Could you check a few things on this model? Use its own coordinates, in mm. Coordinates: 2 decimals unless noted, no trailing zeros. Loops run counter-clockwise (first coordinate to the right, second up) from the corner with the lowest first, then second, coordinate; pieces in that order, holes last. Notation, with made-up numbers: (45, -19.75) - (104, -19.75) arc R19 cw to (104, -15.75) - close; hole circle Ø2 at (67.5, -17). An arc over 180 degrees is marked (long way). One line per question, with ' | ' between items. Start each with the question number.
1. I want a section at A-A, the plane y = -55. Write out the boundary of the cut face in (x, z).
2. I want a section at B-B, the plane x = 20.5. Write out the boundary of the cut face in (y, z), then the cut area to 3 significant figures.
3. I want a section at D-D, the plane y = -79.5. Write out the boundary of the cut face in (x, z).
4. Please list where these lines run through material, in increasing order: L1, parallel to Z at x = -4, y = -69.5; L2, parallel to X at y = -117.5, z = -1; L3, parallel to X at y = -47, z = -3.5. Write a range as [from, to].
5. I'm going to push flat-ended pins straight in: P1, Ø12, axis at x = -25.5, y = -16, coming from the +Z side; P2, Ø1.5, axis at y = -92.5, z = -15, coming from the -X side; P3, Ø4.5, axis at y = -27.5, z = -28, coming from the +X side. Where does each tip first touch, or does it pass through?
6. I want a section at C-C, the plane z = -20. Write out the boundary of the cut face in (x, y).
from build123d import *

# Parameters (mm, degrees)
F1_DEPTH = 130
F3_DEPTH = 38


with BuildPart() as f1:
    # F0 (on Front) → F1 (new body)
    with BuildSketch(Plane.XZ):
        with BuildLine():
            ThreePointArc((39.633115, 3.448032), (1.680451, -18.731595), (-40.366885, -31.551968))
            Line((-40.366885, -31.551968), (39.633115, -31.551968))
            Line((39.633115, -31.551968), (39.633115, 3.448032))
        make_face()
    extrude(amount=F1_DEPTH)

    # F2 (on face) → F3 (cut)
    with BuildSketch(Plane.YZ.offset(39.633115)):
        Polygon((-117.5, -22.891714), (-122.5, -31.551968), (-112.5, -31.551968), align=None)
        Polygon((-102.5, -22.891714), (-107.5, -31.551968), (-97.5, -31.551968), align=None)
        Polygon((-87.5, -22.891714), (-92.5, -31.551968), (-82.5, -31.551968), align=None)
        Polygon((-72.5, -22.891714), (-77.5, -31.551968), (-67.5, -31.551968), align=None)
        Polygon((-57.5, -22.891714), (-62.5, -31.551968), (-52.5, -31.551968), align=None)
        Polygon((-47.5, -31.551968), (-37.5, -31.551968), (-42.5, -22.891714), align=None)
        Polygon((-32.5, -31.551968), (-22.5, -31.551968), (-27.5, -22.891714), align=None)
        Polygon((-17.5, -31.551968), (-7.5, -31.551968), (-12.5, -22.891714), align=None)
    extrude(amount=-F3_DEPTH, mode=Mode.SUBTRACT)


solid = f1.part
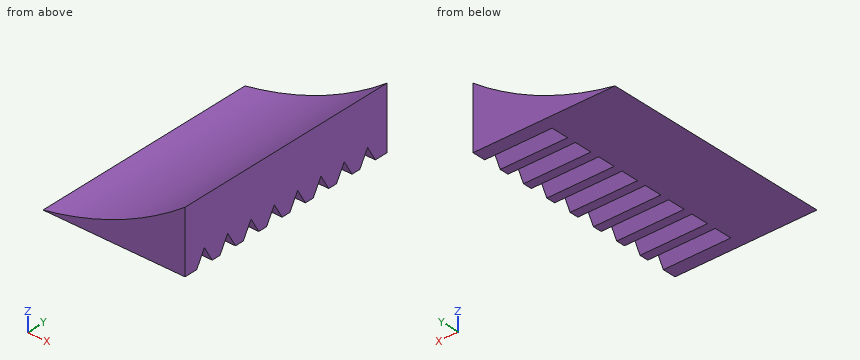
Results are:
1) outline: (-40.37, -31.55) - (1.63, -31.55) - (1.63, -27.22) - (39.63, -27.22) - (39.63, 3.45) arc R189.15 cw to start
2) outline: (-130, -31.55) - (-122.5, -31.55) - (-117.5, -22.89) - (-112.5, -31.55) - (-107.5, -31.55) - (-102.5, -22.89) - (-97.5, -31.55) - (-92.5, -31.55) - (-87.5, -22.89) - (-82.5, -31.55) - (-77.5, -31.55) - (-72.5, -22.89) - (-67.5, -31.55) - (-62.5, -31.55) - (-57.5, -22.89) - (-52.5, -31.55) - (-47.5, -31.55) - (-42.5, -22.89) - (-37.5, -31.55) - (-32.5, -31.55) - (-27.5, -22.89) - (-22.5, -31.55) - (-17.5, -31.55) - (-12.5, -22.89) - (-7.5, -31.55) - (0, -31.55) - (0, -9.21) - (-130, -9.21) - close | area: 2,560 mm2
3) outline: (-40.37, -31.55) - (39.63, -31.55) - (39.63, 3.45) arc R189.15 cw to start
4) L1: z = [-31.55, -21.11] | L2: x = [33.47, 39.63] | L3: x = [29.76, 39.63]
5) P1: stops at z = -26.53 | P2: stops at x = 8.16 | P3: stops at x = 1.63
6) outline: (-1.29, -130) - (39.63, -130) - (39.63, 0) - (-1.29, 0) - close
